Here's how the part is built. I have some questions about the finished solid (model axes, mm). A direction names the side the tool comes from. Round coordinates to 2 decimals unless told otherwise and drop trailing zeros. Loops run counter-clockwise (first coordinate to the right, second up) from the corner with the lowest first, then second, coordinate; pieces in that order, holes last. Notation, with made-up numbers: (-18.75, 87) -> (-4.75, 87) arc R25 ccw to (-4.75, 126) -> close; hole circle Ø8 at (-30.75, -15). An arc over 180 degrees is marked (long way). Use one line per item in the form item = value. Start each with the question number.
Item 1: Thinking about a two-plate mould opening in X: for faces 3 (the face through (0, 15, 62)), 4 (the face through (0, 13, 62)), 5 (the face through (-13.859, 13.797, 60.925)), which applies, released by +X, released by -X, zero draft, split by the parting line, or undercut?
Item 2: If I drill on L1, parallel to X at y = -4, z = 103.5; L2, parallel to X at y = -1.5, z = 163, over which ranges is the centre line in solid material (lowest first)? Write a range as [from, to].
Item 3: If we section it at C-C (z = 80.5): Write out the boundary of the cut face in (x, y).
Item 4: For faces 1 (the face through (0, -15, 62)), 2 (the face through (13, 0, 71)), which set-ups out of +Z, -Z, +X, -X, +Y, -Y let a thin tool reach every point of the face, with its end or its side?
Item 5: If we section it at A-A (y = 0.75): Write out the boundary of the cut face in (x, z).
Item 6: If we section it at D-D (z = 157): Write out the boundary of the cut face in (x, y).
Item 7: If we section it at B-B (x = 3): Write out the boundary of the cut face in (y, z).
Autodesk Inventor part; units mm, degrees
ref_plane "Plano inicial" through (0, 0, -50) normal (0, 0, 1) x (1, 0, 0)
ref_plane "Plano final" through (0, 0, 175) normal (0, 0, 1) x (1, 0, 0)
ref_plane "Plano de trabalho5" through (-15, 0, 175) normal (0.7071, 0, 0.7071) x (0.7071, 0, -0.7071)
ref_plane "Plano inicial" through (0, 0, -50) normal (0, 0, 1) x (1, 0, 0)
ref_plane "Plano final" through (0, 0, 175) normal (0, 0, 1) x (1, 0, 0)
sketch "Esboço" plane through (0, 0, 0) normal (0, 0, 1) x (1, 0, 0)
  line L0 (-15, -11) -> (-15, 11)
  line L1 (-11, 15) -> (11, 15)
  line L2 (15, 11) -> (15, -11)
  line L3 (11, -15) -> (-11, -15)
  arc A0 (-15, -11) -> (-11, -15) centre (-11, -11) ccw
  arc A1 (15, 11) -> (11, 15) centre (11, 11) ccw
  arc A2 (-11, 15) -> (-15, 11) centre (-11, 11) ccw
  arc A3 (11, -15) -> (15, -11) centre (11, -11) ccw
  arc A4 (-11, 13) -> (-13, 11) centre (-11, 11) ccw
  line L4 (-11, 13) -> (11, 13)
  arc A5 (13, 11) -> (11, 13) centre (11, 11) ccw
  line L5 (13, 11) -> (13, -11)
  arc A6 (11, -13) -> (13, -11) centre (11, -11) ccw
  line L6 (11, -13) -> (-11, -13)
  arc A7 (-13, -11) -> (-11, -13) centre (-11, -11) ccw
  line L7 (-13, -11) -> (-13, 11)
  line L8 (0, 22.1598) -> (0, -22.1598) construction
  line L9 (-22.1598, 0) -> (22.1598, 0) construction
  dimension "d7" = 4
  dimension "d9" = 30
  dimension "d11" = 30
  dimension "d12" = 2
  dimension "d15" = 15
  dimension "d16" = 15
extrude "Corpo" add sketch "Esboço" along normal up to surface (225 mm away) from surface at -50
sketch "Sketch3" plane through (0, 0, 0) normal (0, 0, 1) x (1, 0, 0)
  line L0 (0, 0) -> (10, 0)
ref_plane "Work Plane3" through (0, 0, 0) normal (0, -1, 0) x (1, 0, 0)
sketch "Sketch4" plane through (0, 0, 0) normal (0, -1, 0) x (1, 0, 0)
  line L0 (-2, -50) -> (12, -50)
  line L1 (-2, 175) -> (12, 175)
  dimension "d18" = 225
ref_plane "Plano de trabalho5" through (-15, 0, 175) normal (0.7071, 0, 0.7071) x (0.7071, 0, -0.7071)
split "Dividir2" plane through (-15, 0, 175) removes the side toward (0.7071, 0, 0.7071)
ref_plane "Plano de trabalho6" through (0, 15, 175) normal (0, 0, 1) x (1, 0, 0)
split "Dividir3" plane through (0, 15, 175) removes the side toward (0, 0, 1)
ref_plane "Plano de trabalho7" through (-15, 2.5, -50) normal (0.8575, 0, -0.5145) x (-0.5145, 0, -0.8575)
split "Dividir4" plane through (-15, 2.5, -50) removes the side toward (0.8575, 0, -0.5145)
equation "\"d7\" = G_IR"
equation "\"d9\" = G_W"
equation "\"d11\" = G_H"
equation "\"d12\" = G_T"
equation "\"d15\" = 0.5 * d9"
equation "\"d16\" = 0.5 * d11"
equation "\"d3\" = G_L"
equation "\"G_W\" = 30"
equation "\"G_H\" = 30"
equation "\"G_T\" = 2"
equation "\"G_IR\" = 4"
equation "\"G_L\" = d18"
equation "\"G_OFFSET_END\" = 0"
equation "\"d14\" = G_OFFSET_END + B_L"
equation "\"B_L\" = 175"
properties part number "ISO 10799-2 - 30x30x2 - 225" material "Aço, suave"
Values found:
q1.face_3 = zero draft
q1.face_4 = undercut
q1.face_5 = released by -X
q2.L1 = [-15, -13], [13, 15]
q2.L2 = [-15, -13]
q3.outline = (-15, -11) arc R4 ccw to (-11, -15) -> (11, -15) arc R4 ccw to (15, -11) -> (15, 11) arc R4 ccw to (11, 15) -> (-11, 15) arc R4 ccw to (-15, 11) -> close; hole (-13, -11) arc R2 ccw to (-11, -13) -> (11, -13) arc R2 ccw to (13, -11) -> (13, 11) arc R2 ccw to (11, 13) -> (-11, 13) arc R2 ccw to (-13, 11) -> close
q4.face_1 = +Z, -Z, +X, -X, -Y
q4.face_2 = +Z, -Z
q5.outline = (-15, -50) -> (-13, -46.67) -> (-13, 173) -> (-15, 175) -> close; (13, -3.33) -> (15, 0) -> (15, 145) -> (13, 147) -> close
q6.outline = (-15, -11) arc R4 ccw to (-11, -15) -> (3, -15) -> (3, -13) -> (-11, -13) arc R2 cw to (-13, -11) -> (-13, 11) arc R2 cw to (-11, 13) -> (3, 13) -> (3, 15) -> (-11, 15) arc R4 ccw to (-15, 11) -> close
q7.outline = (-15, -20) -> (-13, -20) -> (-13, 157) -> (-15, 157) -> close; (13, -20) -> (15, -20) -> (15, 157) -> (13, 157) -> close
